Could you check a few things on this model? Use its own coordinates, in mm. A direction names the side the tool comes from. Give positions to 0.01 mm unless a question says otherwise; leave off trailing zeros. Write each loop counter-clockwise with the first axis right and the second up, starting at its lowest first coordinate (ties: lowest second). Pieces come first, ordered by that corner, then holes. Notation, with made-up numbers: (-22.75, 89.5) - (5.25, 89.5) arc R15 cw to (5.25, 104.5) - close; hole circle Ø9 at (33, -13). An arc over 180 degrees is marked (long way). Answer in a Markdown table with one row per item.
Autodesk Inventor part; units mm, degrees
ref_plane "YZ Plane" through (0, 0, 0) normal (1, 0, 0) x (0, 1, 0)
ref_plane "XZ Plane" through (0, 0, 0) normal (0, 1, 0) x (-1, 0, 0)
ref_plane "XY Plane" through (0, 0, 0) normal (0, 0, 1) x (1, 0, 0)
sketch "Sketch1" plane through (0, 0, 0) normal (0, 0, 1) x (1, 0, 0)
  line L0 (-10, 3.25) -> (10, 3.25)
  line L1 (10, 3.25) -> (10, -3.25)
  line L2 (10, -3.25) -> (-10, -3.25)
  line L3 (-10, -3.25) -> (-10, 3.25)
  line L4 (-10, 3.25) -> (10, -3.25) construction
  line L5 (10, 3.25) -> (-10, -3.25) construction
  point P0 (0, 0)
  dimension "d0" = 20
  dimension "d1" = 6.5
extrude "Extrusion1" add sketch "Sketch1" along normal blind 1.6
sketch "Sketch2" plane through (0, 0, 1.6) normal (0, 0, 1) x (1, 0, 0)
  line L0 (10, -3.25) -> (10, 3.25)
  line L1 (-10, 3.25) -> (-10, -3.25)
  line L2 (10, 3.25) -> (-10, 3.25)
  point P0 (0, 0)
  point P1 (-8, 0)
  point P2 (8, 0)
  dimension "d4" = 2
  dimension "d5" = 2
  dimension "d6" = 3.25
  dimension "d7" = 3.25
hole "Hole1" at (-8, 0, 1.6) at (8, 0, 1.6) direction (0, 0, -1) diameter 2.1 end through all
sketch "Sketch3" plane through (0, 0, 1.6) normal (0, 0, 1) x (1, 0, 0)
  line L0 (-3.37, 1.68) -> (3.37, 1.68)
  line L1 (4.57, 0.48) -> (4.57, -0.48)
  line L2 (3.37, -1.68) -> (-3.37, -1.68)
  line L3 (-4.57, -0.48) -> (-4.57, 0.48)
  line L4 (-4.57, 1.68) -> (4.57, -1.68) construction
  line L5 (4.57, 1.68) -> (-4.57, -1.68) construction
  arc A0 (-3.37, 1.68) -> (-4.57, 0.48) centre (-3.37, 0.48) ccw
  arc A1 (4.57, 0.48) -> (3.37, 1.68) centre (3.37, 0.48) ccw
  arc A2 (3.37, -1.68) -> (4.57, -0.48) centre (3.37, -0.48) ccw
  arc A3 (-4.57, -0.48) -> (-3.37, -1.68) centre (-3.37, -0.48) ccw
  point P0 (0, 0)
  point P1 (-4.57, 0)
  point P2 (4.57, 0)
  dimension "d15" = 9.14
  dimension "d16" = 3.36
  dimension "d17" = 1.2
extrude "Extrusion2" cut sketch "Sketch3" against normal blind 1.6
properties part number "USB-C_face_plate"
1) Imagine slicing it at B-B (z = 0.55). List the corners of the cut face in (x, y) for me.
Check values:
| item | result |
|---|---|
| outline | (-10, -3.25) - (10, -3.25) - (10, 3.25) - (-10, 3.25) - close; hole circle Ø2.1 at (-8, 0); hole (-4.57, -0.48) arc R1.2 ccw to (-3.37, -1.68) - (3.37, -1.68) arc R1.2 ccw to (4.57, -0.48) - (4.57, 0.48) arc R1.2 ccw to (3.37, 1.68) - (-3.37, 1.68) arc R1.2 ccw to (-4.57, 0.48) - close; hole circle Ø2.1 at (8, 0) |
2) On a 3-axis mill with a long thin cutter (end or side, diameter ignored), from which of +Z, -Z, +X, -X, +Y, -Y can I reach the whole of each face in a straight line? I mean faces 5 (the face through (-10, 0, 1)), 6 (the face through (4.57, 0, 1)). Say none if no direction works.
Check values:
| item | result |
|---|---|
| face 5 | +Z, -Z, -X, +Y, -Y |
| face 6 | +Z, -Z |
3) Imagine slicing it at D-D (x = 8). List the corners of the cut face in (y, z) for me.
Check values:
| item | result |
|---|---|
| outline | (-3.25, 0) - (-1.05, 0) - (-1.05, 1.6) - (-3.25, 1.6) - close; (1.05, 0) - (3.25, 0) - (3.25, 1.6) - (1.05, 1.6) - close |
4) Imagine slicing it at A-A (x = 0.25). List the corners of the cut face in (y, z) for me, then the cut area to 3 significant figures.
Check values:
| item | result |
|---|---|
| outline | (-3.25, 0) - (-1.68, 0) - (-1.68, 1.6) - (-3.25, 1.6) - close; (1.68, 0) - (3.25, 0) - (3.25, 1.6) - (1.68, 1.6) - close |
| area | 5.02 mm2 |
5) We'd pull the mould along Y, two halves only. Please class faces 1 (the face through (0, 2, 1.6)), 2 (the face through (4.228, 1.319, 0.811)), 3 (the face through (0, 3.25, 1)), 4 (the face through (6.96, 0.14, 0.79)): +Y half, -Y half, draft (parallel to the pull), parting line (faces both ways), or undercut.
Check values:
| item | result |
|---|---|
| face 1 | draft |
| face 2 | undercut |
| face 3 | +Y half |
| face 4 | undercut |
6) Will this pin go through, and if not, where does the flat tip stop? P1, Ø3, axis at x = -4, y = 0, coming from the -Z side.
Check values:
| item | result |
|---|---|
| P1 | stops at z = 0 |
7) Imagine slicing it at C-C (y = 0). List the corners of the cut face in (x, z) for me, then the cut area to 3 significant figures.
Check values:
| item | result |
|---|---|
| outline | (-10, 0) - (-9.05, 0) - (-9.05, 1.6) - (-10, 1.6) - close; (-6.95, 0) - (-4.57, 0) - (-4.57, 1.6) - (-6.95, 1.6) - close; (4.57, 0) - (6.95, 0) - (6.95, 1.6) - (4.57, 1.6) - close; (9.05, 0) - (10, 0) - (10, 1.6) - (9.05, 1.6) - close |
| area | 10.7 mm2 |
8) If I drill on line 1 (X direction, y = 0, z = 0.7); line 2 (Y direction, x = -8, z = 0.8); line 3 (X direction, y = 0.75, z = 1.3), over which ranges is the centre line in solid material (lowest first)?
Check values:
| item | result |
|---|---|
| line 1 | x = -10 to -9.05, -6.95 to -4.57, 4.57 to 6.95, 9.05 to 10 |
| line 2 | y = -3.25 to -1.05, 1.05 to 3.25 |
| line 3 | x = -10 to -8.73, -7.27 to -4.54, 4.54 to 7.27, 8.73 to 10 |
